```python
from build123d import *

# Parameters (mm, degrees)
EXTRUDE1_DEPTH                    = 36.195
SKETCH17_W                        = 99.9998
SKETCH17_H                        = 10.668
EXTRUDE4_DEPTH                    = 17.145
CUT_EXTRUDE2_DEPTH                = 73.39
SKETCH19_W                        = 99.9998
SKETCH19_H                        = 9.652
CUT_EXTRUDE3_DEPTH                = 86.2
F_1_4_20_TAPPED_HOLE1_D           = 5.1054
F_1_4_20_TAPPED_HOLE1_DEPTH       = 22.86
F_1_4_20_TAPPED_HOLE1_CBORE_D     = 6.35
F_1_4_20_TAPPED_HOLE1_CBORE_DEPTH = 19.05
F_1_4_20_TAPPED_HOLE1_TIP         = 1.533816902
CHAMFER1_SIZE                     = 2.54
SKETCH24_R                        = 3.9878
EXTRUDE5_DEPTH                    = 6.35
CHAMFER3_SIZE                     = 6.35


with BuildPart() as part:
    # Sketch5 → Extrude1 (new body)
    with BuildSketch(Plane.XY):
        with BuildLine():
            Line((48.9458, -36.195), (48.9458, 36.195))
            Line((48.9458, 36.195), (-51.054, 36.195))
            Line((-51.054, 36.195), (-51.054, 23.8125))
            Line((-51.054, 23.8125), (-34.544, 23.8125))
            ThreePointArc((-34.544, 23.8125), (-10.7315, 0), (-34.544, -23.8125))
            Line((-34.544, -23.8125), (-51.054, -23.8125))
            Line((-51.054, -23.8125), (-51.054, -36.195))
            Line((-51.054, -36.195), (48.9458, -36.195))
        make_face()
    extrude(amount=EXTRUDE1_DEPTH)

    # Sketch17 → Extrude4 (add)
    with BuildSketch(Plane.XY.offset(36.195)):
        with Locations((-1.0541, 30.861)):
            Rectangle(SKETCH17_W, SKETCH17_H)
        with Locations((-1.0541, -30.861)):
            Rectangle(SKETCH17_W, SKETCH17_H)
    extrude(amount=EXTRUDE4_DEPTH)

    # Sketch16 → Cut-Extrude2 (cut, through all)
    with BuildSketch(Plane.XZ.offset(36.195)):
        with BuildLine():
            Line((-25.6286, 50.8), (-25.6286, 53.34))
            Line((-25.6286, 53.34), (-38.3794, 53.34))
            Line((-38.3794, 53.34), (-38.3794, 50.8))
            ThreePointArc((-38.3794, 50.8), (-32.004, 44.4246), (-25.6286, 50.8))
        make_face()
        with BuildLine():
            Line((31.5087, 50.8), (31.5087, 53.34))
            Line((31.5087, 53.34), (18.7833, 53.34))
            Line((18.7833, 53.34), (18.7833, 50.8))
            ThreePointArc((18.7833, 50.8), (25.146, 44.4373), (31.5087, 50.8))
        make_face()
    extrude(amount=-CUT_EXTRUDE2_DEPTH, mode=Mode.SUBTRACT)

    # Sketch19 → Cut-Extrude3 (cut)
    with BuildSketch(Plane.XZ.offset(36.195)):
        with Locations((-1.0541, 4.826)):
            Rectangle(SKETCH19_W, SKETCH19_H)
    extrude(amount=-CUT_EXTRUDE3_DEPTH, mode=Mode.SUBTRACT)

    # 1_4-20 Tapped Hole1
    with Locations(Plane(origin=(0, 0, 9.652), x_dir=(-1, 0, 0), z_dir=(0, 0, -1))):
        with Locations((7.874, 26.9875), (7.874, -26.9875)):
            CounterBoreHole(F_1_4_20_TAPPED_HOLE1_D / 2, F_1_4_20_TAPPED_HOLE1_CBORE_D / 2, F_1_4_20_TAPPED_HOLE1_CBORE_DEPTH, depth=F_1_4_20_TAPPED_HOLE1_DEPTH)
            with Locations((0, 0, -(F_1_4_20_TAPPED_HOLE1_DEPTH + F_1_4_20_TAPPED_HOLE1_TIP / 2))):  # 118° drill point
                Cone(0, F_1_4_20_TAPPED_HOLE1_D / 2, F_1_4_20_TAPPED_HOLE1_TIP, mode=Mode.SUBTRACT)

    # Chamfer1
    chamfer1_edges = [part.edges().sort_by_distance(p)[0] for p in [
        (-51.054, -23.8125, 22.9235),
        (-51.054, 23.8125, 22.9235),
        (-51.054, -36.195, 31.496),
        (-51.054, 36.195, 31.496),
    ]]
    chamfer(chamfer1_edges, length=CHAMFER1_SIZE)

    # Sketch24 → Extrude5 (cut)
    with BuildSketch(Plane(origin=(0, 0, 9.652), x_dir=(-1, 0, 0), z_dir=(0, 0, -1))):
        with Locations((7.874, -26.9875)):
            Circle(SKETCH24_R)
        with Locations((7.874, 26.9875)):
            Circle(SKETCH24_R)
    extrude(amount=-EXTRUDE5_DEPTH, mode=Mode.SUBTRACT)

    # Chamfer3
    chamfer3_edges = [part.edges().sort_by_distance(p)[0] for p in [
        (-51.054, -30.00375, 53.34),
        (-51.054, 30.00375, 53.34),
    ]]
    chamfer(chamfer3_edges, length=CHAMFER3_SIZE)


solid = part.part
```
Could you check a few things on this model? Use its own coordinates, in mm. A direction names the side the tool comes from. Give positions to 0.01 mm unless a question says otherwise; leave off trailing zeros. Loops run counter-clockwise (first coordinate to the right, second up) from the corner with the lowest first, then second, coordinate; pieces in that order, holes last. Notation, with made-up numbers: (9, 62.25) -> (45, 62.25) arc R33 cw to (45, 96.25) -> close; hole circle Ø3 at (58, 17). An arc over 180 degrees is marked (long way). Put each result on its own line as item: value.
(1) Imagine slicing it at D-D on y = -11.5. Write out the boundary of the cut face in (x, z) (1 decimal), plus the area to 3 significant figures.
Computed:
outline: (-13.7, 9.7) -> (48.9, 9.7) -> (48.9, 36.2) -> (-13.7, 36.2) -> close
area: 1,660 mm^2
(2) Please list where these lines run through material, in increasing order: probe 1 along Y at (x, z) = (-43, 32) (1 decimal); probe 2 along Y at (x, z) = (-19, 42.5) (3 decimals); probe 3 along Z at (x, y) = (-18, 17.5) (3 decimals). Write a range as [from, to].
Computed:
probe 1: [-36.2, -23.8], [23.8, 36.2]
probe 2: [-36.195, -25.527], [25.527, 36.195]
probe 3: [9.652, 36.195]
(3) Imagine slicing it at C-C on y = 0. Write out the boundary of the cut face in (x, z) (1 decimal), plus the area to 3 significant figures.
Computed:
outline: (-10.7, 9.7) -> (48.9, 9.7) -> (48.9, 36.2) -> (-10.7, 36.2) -> close
area: 1,580 mm^2
(4) Imagine slicing it at A-A on x = 4.5. Write out the boundary of the cut face in (y, z) (3 decimals), plus the area to 3 significant figures.
Computed:
outline: (-36.195, 9.652) -> (36.195, 9.652) -> (36.195, 53.34) -> (25.527, 53.34) -> (25.527, 36.195) -> (-25.527, 36.195) -> (-25.527, 53.34) -> (-36.195, 53.34) -> close
area: 2,290 mm^2
(5) For faces 1 (the face through (-25.629, 31, 52)), 2 (the face through (0, 36.195, 31)), 3 (the face through (-41, -23.812, 23)), 4 (the face through (-8.206, -24.457, 30.634)), 5 (the face through (40, -31, 53.34)), which set-ups out of +Z, -Z, +X, -X, +Y, -Y let a thin tool reach every point of the face, with its end or its side?
Computed:
face 1: +Z, +Y, -Y
face 2: +Z, -Z, +X, -X, +Y
face 3: +Z, -Z, -X
face 4: -Z
face 5: +Z, +X, -X, +Y, -Y
(6) I'm going to push flat-ended pins straight in: pin 1 Ø4 at (x, y) = (-8, 25.5) entering from -Z; pin 2 Ø10 at (x, y) = (-7.87, -26.99) entering from -Z; pin 3 Ø3 at (y, z) = (-20.5, 36.5) entering from -X; pin 4 Ø6 at (y, z) = (3.5, 40.5) entering from +X. Where does each tip first touch, or does it pass through?
Computed:
pin 1: z = 16
pin 2: z = 9.65
pin 3: x = -25.36
pin 4: through
(7) Thinking about a two-plate mould opening in X: for faces 6 (the face through (-51.054, 30, 28)), 7 (the face through (48.946, -1, 26)), 8 (the face through (-42, -31, 53.34)), 9 (the face through (-38.379, 31, 52)), which applies, pulls with the +X half, pulls with the -X half, needs draft (parallel to the pull), parting line crosses it, or undercut?
Computed:
face 6: pulls with the -X half
face 7: pulls with the +X half
face 8: needs draft
face 9: undercut
(8) Imagine slicing it at B-B on z = 21. State how many separate pieces and enclosed holes the cut face has, plus the area to 3 significant figures.
Computed:
separate pieces: 1
enclosed holes: 2
area: 5,490 mm^2
